```python
from build123d import *

# Parameters (mm, degrees)
BOSS_EXTRUDE1_DEPTH     = 5
CUT_EXTRUDE1_DEPTH      = 1
CUT_EXTRUDE1_DEPTH_BACK = 6


with BuildPart() as part:
    # Sketch3 → Boss-Extrude1 (new body)
    with BuildSketch(Plane.XY.offset(-218)):
        Polygon((-331.826668729, 452.47886283), (-275.647209147, 408.586658554), (-300.273668161, 377.066228409), (-386.557905491, 444.47886283), (-427.432442284, 444.47886283), (-447.432442284, 460.10457536), (-447.432442284, 561.679955314), (-427.432442284, 561.679955314), (-427.432442284, 452.47886283), align=None)
    extrude(amount=-BOSS_EXTRUDE1_DEPTH)

    # Sketch4 → Cut-Extrude1 (cut, two sides)
    with BuildSketch(Plane(origin=(0, 0, -223), x_dir=(-1, 0, 0), z_dir=(0, 0, -1))) as cut_extrude1_sk:
        Polygon((296.647620515, 424.993978106), (299.95726568, 427.579756302), (302.419911581, 424.427713288), (303.995933089, 425.659036238), (305.71978522, 423.452606128), (304.143763712, 422.221283178), (310.300378466, 414.341175642), (306.990733301, 411.755397445), (300.834118547, 419.635504981), (299.25809704, 418.404182031), (297.534244909, 420.610612141), (299.110266416, 421.841935091), align=None)
        Polygon((309.979258098, 430.333722067), (308.40323659, 429.102399116), (310.127088721, 426.895969006), (311.703110229, 428.127291957), (317.859724982, 420.24718442), (321.169370147, 422.832962617), (315.012755394, 430.713070153), (316.588776901, 431.944393104), (314.86492477, 434.150823214), (313.288903263, 432.919500263), (310.826257361, 436.071543277), (307.516612196, 433.485765081), align=None)
    extrude(amount=CUT_EXTRUDE1_DEPTH, mode=Mode.SUBTRACT)
    extrude(cut_extrude1_sk.sketch, amount=-CUT_EXTRUDE1_DEPTH_BACK, mode=Mode.SUBTRACT)


solid = part.part
```
Geometry check sheet. Reference: the model listing, model coordinates, mm. A direction names the side the tool comes from. Give positions to 0.01 mm unless a question says otherwise; leave off trailing zeros. Loops run counter-clockwise (first coordinate to the right, second up) from the corner with the lowest first, then second, coordinate; pieces in that order, holes last. Notation, with made-up numbers: M -34.5,-11 L -4.5,-11 A17 cw -4.5,4 Z; hole C -4,51 d7. An arc over 180 degrees is marked long. Write item = value, one per line. Start each with the question number.
1. Section check C-C, the plane y = 487.5. Enter the section's corners in (x, z).
2. Section check B-B, the plane x = -414. Enter the section's corners in (y, z).
3. Go/stop test with flat-tipped pins: P1, Ø1, axis at y = 526, z = -220.5, coming from the +X side; P2, Ø2, axis at x = -321, z = -219, coming from the +Y side; P3, Ø1.5, axis at y = 406, z = -221, coming from the +X side. Record where each tip stops, or that it passes through.
4. Thickness scan on probe 1 along X at (y, z) = (420.5, -222.45); probe 2 along X at (y, z) = (543, -218.35); probe 3 along Y at (x, z) = (-406, -219.4). Record the ranges inside material, lowest first.
5. Tool access check on faces 1 (the face through (-427.432, 508, -220)), 2 (the face through (-314.74, 424.24, -220.54)), 3 (the face through (-447.432, 510, -220)), 4 (the face through (-407, 444.479, -220)). Record the directions out of +Z, -Z, +X, -X, +Y, -Y that give a thin tool (end or side, any length) a straight path to the whole face; none if there is none.
6. Draft check along Y on faces 5 (the face through (-287.788, 393.047, -220.465)), 6 (the face through (-307.179, 418.336, -220.535)), 7 (the face through (-303.956, 415.64, -220.535)), 8 (the face through (-303.79, 430.574, -220.465)). Enter one of: +Y half, -Y half, draft (parallel to the pull), parting line (faces both ways), or undercut.
Values follow:
q1.outline = M -447.43,-223 L -427.43,-223 L -427.43,-218 L -447.43,-218 Z
q2.outline = M 444.48,-223 L 452.48,-223 L 452.48,-218 L 444.48,-218 Z
q3.P1 = -427.43
q3.P2 = 444.8
q3.P3 = -277.08
q4.probe_1 = -355.87 to -318.18, -317.66 to -305.49, -297.62 to -290.9
q4.probe_2 = -447.43 to -427.43
q4.probe_3 = 444.48 to 452.48
q5.face_1 = +Z, -Z, +X, +Y
q5.face_2 = +Z, -Z
q5.face_3 = +Z, -Z, -X, +Y, -Y
q5.face_4 = +Z, -Z, -X, -Y
q6.face_5 = -Y half
q6.face_6 = undercut
q6.face_7 = undercut
q6.face_8 = +Y half
